```python
from build123d import *

# Parameters (mm, degrees)
SKIZZE1_R                       = 9
AUFSATZ_LINEAR_AUSTRAGEN1_DEPTH = 2
SKIZZE3_W                       = 2
SKIZZE3_H                       = 2
SCHNITT_LINEAR_AUSTRAGEN1_DEPTH = 3
SKIZZE4_R                       = 1
SCHNITT_LINEAR_AUSTRAGEN2_DEPTH = 3
KREISMUSTER1_COUNT              = 16


with BuildPart() as part:
    # Skizze1 → Aufsatz-Linear austragen1 (new body)
    with BuildSketch(Plane(origin=(0, 0, 0), x_dir=(1, 0, 0), z_dir=(0, 1, 0))):
        Circle(SKIZZE1_R)
    extrude(amount=AUFSATZ_LINEAR_AUSTRAGEN1_DEPTH)

    # Skizze3 → Schnitt-Linear austragen1 (cut)
    with BuildSketch(Plane(origin=(0, 2, 0), x_dir=(1, 0, 0), z_dir=(0, 1, 0))):
        with Locations((0.014205659, 0.027357499)):
            Rectangle(SKIZZE3_W, SKIZZE3_H)
    extrude(amount=-SCHNITT_LINEAR_AUSTRAGEN1_DEPTH, mode=Mode.SUBTRACT)

    # Skizze4 → Schnitt-Linear austragen2 (cut)
    with BuildSketch(Plane(origin=(0, 2, 0), x_dir=(1, 0, 0), z_dir=(0, 1, 0))):
        with Locations((7.817951829, -0.164692324)):
            Circle(SKIZZE4_R)
    schnitt_linear_austragen2 = extrude(amount=-SCHNITT_LINEAR_AUSTRAGEN2_DEPTH, mode=Mode.SUBTRACT)

    # Kreismuster1: Schnitt-Linear austragen2 ×16 about axis
    kreismuster1_axis = Axis((0, 0, 0), (0, 1, 0))
    for i in range(1, KREISMUSTER1_COUNT):
        add(schnitt_linear_austragen2.rotate(kreismuster1_axis, i * 360 / KREISMUSTER1_COUNT), mode=Mode.SUBTRACT)


solid = part.part
```
Geometry: final body of the model. Coordinates: model frame, mm. A direction names the side the tool comes from. Coordinates: 2 decimals unless noted, no trailing zeros. Order: outer loops, then holes, each group sorted by start corner. A loop starts at its lowest first (then second) coordinate and runs counter-clockwise, first axis right, second up. Notation, with made-up numbers: (51.25, 31.5) - (71.25, 31.5) arc R19 cw to (71.25, 51.5) - close; hole circle Ø8 at (48.5, 18). An arc over 180 degrees is marked (long way). Return JSON: item names as keys, results as strings. Group by question number.
1. Material intervals for line 1 along Z through (x, y) = (-7.25, 1.1); line 2 along X through (y, z) = (1.05, -5.25), sorted ascending. Write a range as [from, to].
2. Set-up query: faces 4 (the face through (0, 1, 0.973)), 5 (the face through (0, 0, 2)). Return all of +Z, -Z, +X, -X, +Y, -Y with unobstructed straight access to the full face (end or side cutting, diameter ignored); none if empty.
3. Cut plane B-B (z = 0.5). Output: boundary loops of the cut face in (x, y), plus the area to 3 significant figures.
4. Cut plane C-C (x = 0.5). Output: boundary loops of the cut face in (y, z).
5. Pull-direction query (Z, two-part tool) for faces 1 (the face through (0, 2, 2)), 2 (the face through (-1.172, 0.986, -8.923)), 3 (the face through (1.014, 1, 0)); classes: pulls with the +Z half, pulls with the -Z half, needs draft (parallel to the pull), parting line crosses it, or undercut.
6. Pin query (flat end, axial travel): pin 1 (1.2 mm diameter, centred on x = 3.14, z = -7.16, fed in from -Y); pin 2 (0.6 mm diameter, centred on y = 0.5, z = -0.5, fed in from -X). Return the tip coordinate at first contact, or that it passes through.
7. Cut plane D-D (y = 0.5). Count the separate pieces of the cut face and the enclosed holes in it, plus the area to 3 significant figures.
8. Cut plane A-A (x = -5.75). Output: boundary loops of the cut face in (y, z).
Resolved:
{
 "1": {"line 1": "z = [-5.33, -4.14], [-2.15, -0.99], [0.66, 1.84], [3.84, 5.33]", "line 2": "x = [-7.31, -6.33], [-4.49, 4.66], [6.63, 7.31]"},
 "2": {"face 4": "+Y, -Y", "face 5": "+Z, -Z, +X, -X, -Y"},
 "3": {"outline": "(-8.99, 0) - (-8.57, 0) - (-8.57, 2) - (-8.99, 2) - close; (-7.07, 0) - (-0.99, 0) - (-0.99, 2) - (-7.07, 2) - close; (1.01, 0) - (6.88, 0) - (6.88, 2) - (1.01, 2) - close; (8.76, 0) - (8.99, 0) - (8.99, 2) - (8.76, 2) - close", "area": "25.2 mm²"},
 "4": {"outline": "(0, -8.99) - (2, -8.99) - (2, -8.76) - (0, -8.76) - close; (0, -6.88) - (2, -6.88) - (2, -1.03) - (0, -1.03) - close; (0, 0.97) - (2, 0.97) - (2, 7.07) - (0, 7.07) - close; (0, 8.57) - (2, 8.57) - (2, 8.99) - (0, 8.99) - close"},
 "5": {"face 1": "needs draft", "face 2": "parting line crosses it", "face 3": "undercut"},
 "6": {"pin 1": "passes through", "pin 2": "stops at x = -9"},
 "7": {"separate pieces": "1", "enclosed holes": "17", "area": "200 mm²"},
 "8": {"outline": "(0, -6.92) - (2, -6.92) - (2, -6.59) - (0, -6.59) - close; (0, -4.7) - (2, -4.7) - (2, 4.42) - (0, 4.42) - close; (0, 6.41) - (2, 6.41) - (2, 6.92) - (0, 6.92) - close"}
}
